Design review of the part shown in the three views and the two pictorial views. Dimensions are in mm from the part's minimum x, y and z. Round coordinates to 2 decimals unless told otherwise and drop trailing zeros. Order: outer loops, then holes, each group sorted by start corner. A loop starts at its lowest first (then second) coordinate and runs counter-clockwise, first axis right, second up. Notation, with made-up numbers: (65.5, 37.5) -> (121.5, 37.5) arc R9 ccw to (121.5, 44.5) -> close; hole circle Ø3 at (3.25, 83.25). An arc over 180 degrees is marked (long way). Put each result on its own line as item: value. Start each with the question number.
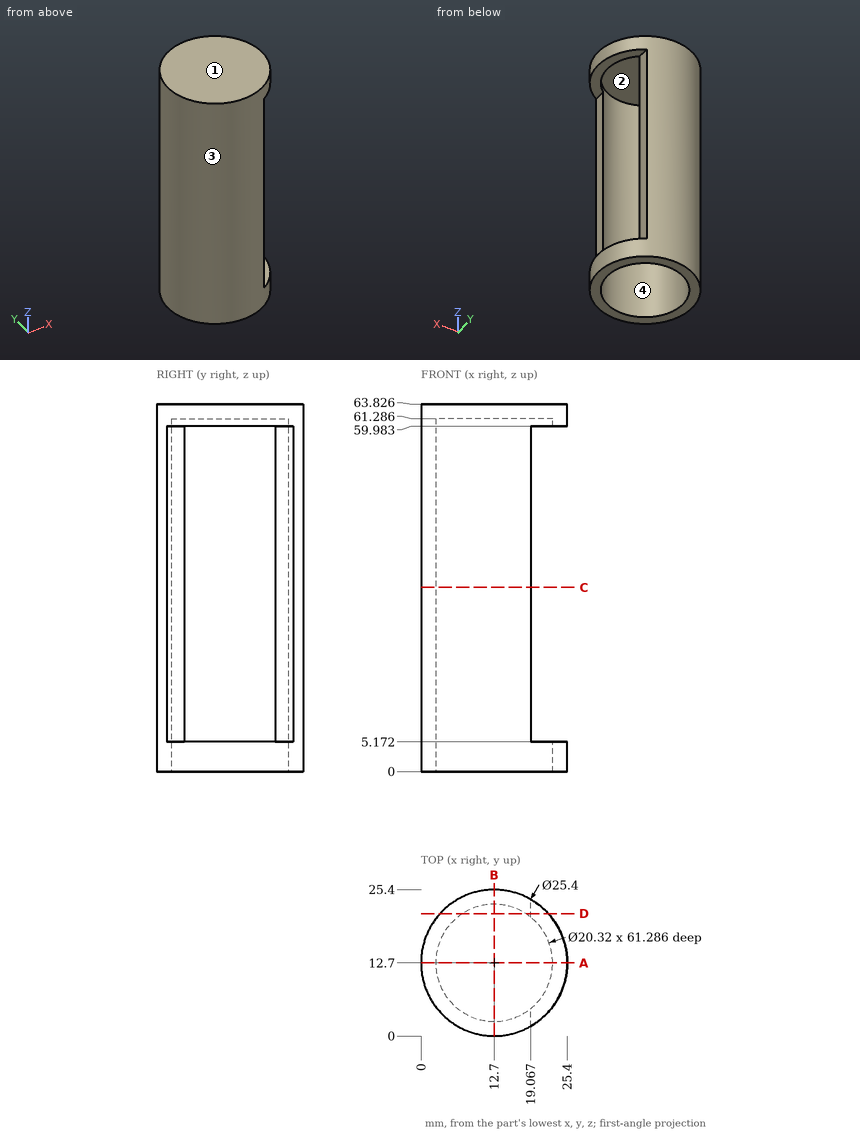
Q1. Draft analysis for pull direction X (two halves, no side actions). For the marked faces 1, 2, 3 and 4, state which applies: +X half, -X half, draft (parallel to the pull), parting line (faces both ways), or undercut.
Q2. Take a section at B-B on x = 12.7. Give the boundary of the cut face in (y, z).
Q3. Take a section at A-A on y = 12.7. Give the boundary of the cut face in (x, z).
Q4. Take a section at C-C on z = 32. Give the boundary of the cut face in (x, y).
Q5. Clearance check with flat-ended pins moving along their axes: pin 1 Ø0.9 at (y, z) = (3, 42.5) entering from +X; pin 2 Ø4 at (y, z) = (7, 13) entering from -X; pin 3 Ø5 at (y, z) = (9.5, 54.5) entering from +X. State where each tip first meets the part, or that it passes through.
Q6. Take a section at D-D on y = 21.25. Give the boundary of the cut face in (x, z).
Q7. Wall thickness on probe 1 along Y at (x, z) = (12.7, 14); probe 2 along Z at (x, y) = (24, 10); probe 3 along Z at (x, y) = (10.75, 13.25): over which ranges is each line inside the solid? List them lowest first. Write a range as [from, to].
Calculated:
1. face 1: draft
1. face 2: undercut
1. face 3: parting line
1. face 4: undercut
2. outline: (0, 0) -> (2.54, 0) -> (2.54, 61.29) -> (22.86, 61.29) -> (22.86, 0) -> (25.4, 0) -> (25.4, 63.83) -> (0, 63.83) -> close
3. outline: (0, 0) -> (2.54, 0) -> (2.54, 61.29) -> (22.86, 61.29) -> (22.86, 59.98) -> (25.4, 59.98) -> (25.4, 63.83) -> (0, 63.83) -> close; (22.86, 0) -> (25.4, 0) -> (25.4, 5.17) -> (22.86, 5.17) -> close
4. outline: (19.07, 1.71) -> (19.07, 4.78) arc R10.16 cw (long way) to (19.07, 20.62) -> (19.07, 23.69) arc R12.7 ccw (long way) to start
5. pin 1: stops at x = 19.07
5. pin 2: stops at x = 0.55
5. pin 3: stops at x = 4.29
6. outline: (3.31, 0) -> (7.21, 0) -> (7.21, 61.29) -> (18.19, 61.29) -> (18.19, 0) -> (22.09, 0) -> (22.09, 5.17) -> (19.07, 5.17) -> (19.07, 59.98) -> (22.09, 59.98) -> (22.09, 63.83) -> (3.31, 63.83) -> close
7. probe 1: y = [0, 2.54], [22.86, 25.4]
7. probe 2: z = [0, 5.17], [59.98, 63.83]
7. probe 3: z = [61.29, 63.83]
